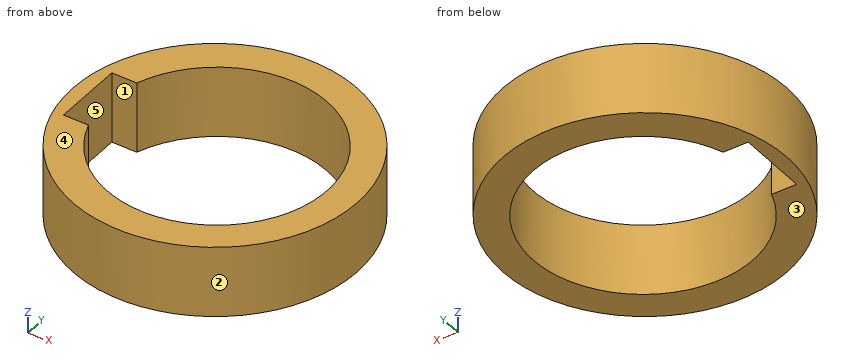
```python
from build123d import *

# Parameters (mm, degrees)
F1_R     = 10
F2_DEPTH = 5
F0_R     = 7.75
F3_DEPTH = 25.4
F4_W     = 8.958675
F4_H     = 5
F5_DEPTH = 80


with BuildPart() as f2:
    # F1 (on Top) → F2 (new body)
    with BuildSketch(Plane.XY):
        Circle(F1_R)
    extrude(amount=F2_DEPTH)

    # F0 (on Top) → F3 (cut)
    with BuildSketch(Plane.XY):
        with Locations((0.138163, 0)):
            Circle(F0_R)
    extrude(amount=F3_DEPTH, mode=Mode.SUBTRACT)

    # F4 (on Top) → F5 (cut)
    with BuildSketch(Plane.XY):
        with Locations((-4.479337, 0)):
            Rectangle(F4_W, F4_H)
    extrude(amount=F5_DEPTH, mode=Mode.SUBTRACT)


solid = f2.part
```
The model under review builds one solid part; all positions refer to its coordinate system, in mm. Face numbers are marked on the shaded views. A direction names the side the tool comes from. Round coordinates to 2 decimals unless told otherwise and drop trailing zeros. Order: outer loops, then holes, each group sorted by start corner. A loop starts at its lowest first (then second) coordinate and runs counter-clockwise, first axis right, second up. Notation, with made-up numbers: (57, 56) -> (75, 56) arc R20 cw to (75, 91) -> close; hole circle Ø9 at (64.25, -23). An arc over 180 degrees is marked (long way). Use a Markdown table: item, result.
Q1. We need section D-D on y = 8.25. Write out the cut boundary in (x, z), then the cut area to 3 significant figures.
Values:
| item | result |
|---|---|
| outline | (-5.65, 0) -> (5.65, 0) -> (5.65, 5) -> (-5.65, 5) -> close |
| area | 56.5 mm^2 |
Q2. We need section B-B on z = 4.3. Write out the cut boundary in (x, y), then the cut area to 3 significant figures.
Values:
| item | result |
|---|---|
| outline | circle Ø20 at (0, 0); hole (-8.96, -2.5) -> (-7.2, -2.5) arc R7.75 ccw (long way) to (-7.2, 2.5) -> (-8.96, 2.5) -> close |
| area | 118 mm^2 |
Q3. For line 1 (Y direction, x = 0.25, z = 3.9); line 2 (X direction, y = -3.75, z = 3.35); line 3 (Y direction, x = 7.25, z = 3.2), list the stretches that pass through material, from the lowest coordinate up.
Values:
| item | result |
|---|---|
| line 1 | y = -10 to -7.75, 7.75 to 10 |
| line 2 | x = -9.27 to -6.64, 6.92 to 9.27 |
| line 3 | y = -6.89 to -3.08, 3.08 to 6.89 |
Q4. Tool access review of the marked faces 4 and 5: name each direction out of +Z, -Z, +X, -X, +Y, -Y from which nothing blocks a thin tool from reaching the whole face with its end or side.
Values:
| item | result |
|---|---|
| face 4 | +Z, +X, -X, +Y, -Y |
| face 5 | +Z, -Z |
Q5. We need section C-C on x = 4.75. Write out the cut boundary in (y, z).
Values:
| item | result |
|---|---|
| outline | (-8.8, 0) -> (-6.23, 0) -> (-6.23, 5) -> (-8.8, 5) -> close; (6.23, 0) -> (8.8, 0) -> (8.8, 5) -> (6.23, 5) -> close |
Q6. Mouldability with a two-part tool opening along X and no side actions: class the marked faces 1, 2 and 3 as +X half, -X half, draft (parallel to the pull), parting line (faces both ways), or undercut.
Values:
| item | result |
|---|---|
| face 1 | undercut |
| face 2 | parting line |
| face 3 | draft |
Q7. Clearance check with flat-ended pins moving along their axes: P1, Ø0.5, axis at x = -8, z = 1.5, coming from the -Y side; P2, Ø4, axis at x = 7.5, y = -2.5, coming from the -Z side; P3, Ø3, axis at y = -5, z = 4, coming from the -X side; P4, Ø0.9, axis at x = -8, z = 2.5, coming from the +Y side. State where each tip first meets the part, or that it passes through.
Values:
| item | result |
|---|---|
| P1 | stops at y = -6.32 |
| P2 | stops at z = 0 |
| P3 | stops at x = -9.37 |
| P4 | stops at y = 6.56 |
Q8. We need section A-A on y = 0. Write out the cut boundary in (x, z).
Values:
| item | result |
|---|---|
| outline | (-10, 0) -> (-8.96, 0) -> (-8.96, 5) -> (-10, 5) -> close; (7.89, 0) -> (10, 0) -> (10, 5) -> (7.89, 5) -> close |
